Work out the finished part from the listing and answer in its coordinate system (mm). Give positions to 0.01 mm unless a question says otherwise; leave off trailing zeros. Loops run counter-clockwise (first coordinate to the right, second up) from the corner with the lowest first, then second, coordinate; pieces in that order, holes last. Notation, with made-up numbers: M 28,21 L 36,21 A19 cw 36,50 Z; hole C 7,-24 d2. An arc over 180 degrees is marked long. Answer in a Markdown table with one row per item. Add a question column.
from build123d import *

# Parameters (mm, degrees)
CYLINDER004_R     = 1.4
CYLINDER004_DEPTH = 61
CYLINDER003_R     = 1.4
CYLINDER003_DEPTH = 10
BOX_W             = 10
BOX_H             = 10
BOX_DEPTH         = 57.5
FILLET_R          = 4
FILLET001_R       = 4


with BuildPart() as cylinder004:
    # Cylinder004 → Cylinder004 (new body)
    with BuildSketch(Plane(origin=(5, 105, -1.5), x_dir=(1, 0, 0), z_dir=(0, 0, 1))):
        Circle(CYLINDER004_R)
    extrude(amount=CYLINDER004_DEPTH)


with BuildPart() as cylinder003:
    # Cylinder003 → Cylinder003 (new body)
    with BuildSketch(Plane(origin=(5, 105, -1), x_dir=(1, 0, 0), z_dir=(0, 0, 1))):
        Circle(CYLINDER003_R)
    extrude(amount=CYLINDER003_DEPTH)


with BuildPart() as spacer:
    # Box → Box (new body)
    with BuildSketch(Plane(origin=(0, 100, 0), x_dir=(1, 0, 0), z_dir=(0, 0, 1))):
        with Locations((5, 5)):
            Rectangle(BOX_W, BOX_H)
    extrude(amount=BOX_DEPTH)

    # Cut003: cut Cylinder003
    add(cylinder003.part, mode=Mode.SUBTRACT)

    # Cut004: cut Cylinder004
    add(cylinder004.part, mode=Mode.SUBTRACT)

    # Fillet
    fillet_edges = [spacer.edges().sort_by_distance(p)[0] for p in [
        (10, 110, 28.75),
    ]]
    fillet(fillet_edges, radius=FILLET_R)

    # Fillet001
    fillet001_edges = [spacer.edges().sort_by_distance(p)[0] for p in [
        (10, 100, 28.75),
    ]]
    fillet(fillet001_edges, radius=FILLET001_R)


solid = spacer.part
(1) Section B-B, the plane z = 39 is taken. Determine the outline of the cut face in (x, y), and give its area (3 significant figures).
(2) Section A-A, the plane x = 5 is taken. Determine the outline of the cut face in (y, z).
(3) Consider line 1 along Y through (x, z) = (5, 36); line 2 along X through (y, z) = (105, 19); line 3 along Y through (x, z) = (5.75, 26). Determine where each line is inside the solid, lowest interval first. Write a range as from..to.
(4) Section D-D, the plane x = 7.75 is taken. Determine the outline of the cut face in (y, z), and give its area (3 significant figures).
(5) Section C-C, the plane y = 105 is taken. Determine the outline of the cut face in (x, z).
Numbers:
| question | item | result |
|---|---|---|
| 1 | outline | M 0,100 L 6,100 A4 ccw 10,104 L 10,106 A4 ccw 6,110 L 0,110 Z; hole C 5,105 d2.8 |
| 1 | area | 87.0 mm² |
| 2 | outline | M 100,0 L 103.6,0 L 103.6,57.5 L 100,57.5 Z; M 106.4,0 L 110,0 L 110,57.5 L 106.4,57.5 Z |
| 3 | line 1 | y = 100..103.6, 106.4..110 |
| 3 | line 2 | x = 0..3.6, 6.4..10 |
| 3 | line 3 | y = 100..103.82, 106.18..110 |
| 4 | outline | M 100.4,0 L 109.6,0 L 109.6,57.5 L 100.4,57.5 Z |
| 4 | area | 529 mm² |
| 5 | outline | M 0,0 L 3.6,0 L 3.6,57.5 L 0,57.5 Z; M 6.4,0 L 10,0 L 10,57.5 L 6.4,57.5 Z |
